```python
from build123d import *

# Parameters (mm, degrees)
SKETCH_W        = 64
SKETCH_H        = 48
PAD_DEPTH       = 1
POCKET_DEPTH    = 1.001
SKETCH002_R     = 2.5
PAD001_DEPTH    = 2.5
SKETCH003_R     = 1.2
POCKET001_DEPTH = 2.5


with BuildPart() as part:
    # Sketch → Pad (new body)
    with BuildSketch(Plane.XY):
        Rectangle(SKETCH_W, SKETCH_H)
    extrude(amount=PAD_DEPTH)

    # Sketch001 → Pocket (cut, through all)
    with BuildSketch(Plane.XY.offset(1)):
        Polygon((-27, 14), (-27, -14), (-22, -14), (-22, -19), (22, -19), (22, -14), (27, -14), (27, 14), (22, 14), (22, 19), (-22, 19), (-22, 14), align=None)
    extrude(amount=-POCKET_DEPTH, mode=Mode.SUBTRACT)

    # Sketch002 → Pad001 (new body)
    with BuildSketch(Plane.XY.offset(1)):
        with Locations((-27.305, 19.05)):
            Circle(SKETCH002_R)
        with Locations((-27.305, -19.05)):
            Circle(SKETCH002_R)
        with Locations((27.305, 19.05)):
            Circle(SKETCH002_R)
        with Locations((27.305, -19.05)):
            Circle(SKETCH002_R)
    extrude(amount=PAD001_DEPTH)

    # Sketch003 → Pocket001 (cut)
    with BuildSketch(Plane.XY.offset(3.5)):
        with Locations((27.305, 19.05)):
            Circle(SKETCH003_R)
        with Locations((-27.305, -19.05)):
            Circle(SKETCH003_R)
        with Locations((27.305, -19.05)):
            Circle(SKETCH003_R)
        with Locations((-27.305, 19.05)):
            Circle(SKETCH003_R)
    extrude(amount=-POCKET001_DEPTH, mode=Mode.SUBTRACT)


solid = part.part
```
Input: part model. Units: mm. Frame: model coordinates. A direction names the side the tool comes from. Give positions to 0.01 mm unless a question says otherwise; leave off trailing zeros. Loops run counter-clockwise (first coordinate to the right, second up) from the corner with the lowest first, then second, coordinate; pieces in that order, holes last.
1) Contact query for a flat-ended pin moving along its axis: pin 1 (24 mm diameter, centred on x = 14.5, y = -10.5, fed in from +Z). Output: stop coordinate, or through.
A:
pin 1: stops at z = 1
2) Mould query, pull axis Y, two halves, no side actions, for faces 1 (the flat face through (26, 20, 3.5)), 2 (the cylindrical face through (24.807, 19.16, 2.232)). Classes: released by +Y, released by -Y, zero draft, split by the parting line, or undercut.
A:
face 1: zero draft
face 2: undercut
3) Section query C-C on x = 24. Return the cut outline in (y, z).
A:
outline: (-24, 0) - (-14, 0) - (-14, 1) - (-24, 1) - close; (14, 0) - (24, 0) - (24, 1) - (14, 1) - close
4) Section query A-A on z = 2.55. Return the cut outline in (x, y) (3 decimals), and give its area (3 significant figures).
A:
outline: circle Ø5 at (-27.305, -19.05); circle Ø5 at (-27.305, 19.05); circle Ø5 at (27.305, -19.05); circle Ø5 at (27.305, 19.05); hole circle Ø2.4 at (-27.305, -19.05); hole circle Ø2.4 at (-27.305, 19.05); hole circle Ø2.4 at (27.305, -19.05); hole circle Ø2.4 at (27.305, 19.05)
area: 60.4 mm2
5) Section query B-B on y = -12.5. Return the cut outline in (x, z).
A:
outline: (-32, 0) - (-27, 0) - (-27, 1) - (-32, 1) - close; (27, 0) - (32, 0) - (32, 1) - (27, 1) - close
6) Reachability of faces 3 (the flat face through (0, -21, 0)), 4 (the flat face through (27, -19, 1)) from +Z, -Z, +X, -X, +Y, -Y: full face, straight path, thin tool, end or side. Return the list, or none.
A:
face 3: -Z, +X, -X, +Y, -Y
face 4: +Z
7) Line query: L1, parallel to Y at x = 26, z = 0.65; L2, parallel to X at y = -10, z = 0.2; L3, parallel to X at y = -20, z = 2.9. Output: solid intervals per line, ascending.
A:
L1: y = -24 to -14, 14 to 24
L2: x = -32 to -27, 27 to 32
L3: x = -29.62 to -28.04, -26.57 to -24.99, 24.99 to 26.57, 28.04 to 29.62
